from build123d import *

# Parameters (mm, degrees)
CUT_EXTRUDE1_REACH             = 92.696
SKETCH3_R                      = 3.571875
CUT_EXTRUDE1_DIRECTION_2_DEPTH = 91.696141042
SKETCH4_R                      = 4.7625
CUT_EXTRUDE2_DEPTH             = 2.54


with BuildPart() as part:
    # Sketch2 → Revolve1 (revolve)
    with BuildSketch(Plane(origin=(0, 0, 0), x_dir=(0, 0, -1), z_dir=(1, 0, 0)), mode=Mode.PRIVATE) as revolve1_sk:
        Polygon((0, 63.5), (0, 60.325), (6.35, 60.325), (6.35, 0), (12.7, 0), (12.7, 63.5), align=None)
    revolve(revolve1_sk.sketch.rotate(Axis((0, 0, 40.533532934), (0, 0, -1)), 90), axis=Axis((0, 0, 40.533532934), (0, 0, -1)))

    # Sketch3 → Cut-Extrude1 (cut, up to next)
    with BuildSketch(Plane(origin=(0, 0, -12.7), x_dir=(-1, 0, 0), z_dir=(0, 0, -1)), mode=Mode.PRIVATE) as cut_extrude1_sk1:
        with Locations(Location((0, 0, 0), (0, 0, 180))):
            Circle(SKETCH3_R)
    cut_extrude1_tool1 = extrude(cut_extrude1_sk1.sketch, amount=-CUT_EXTRUDE1_REACH, mode=Mode.PRIVATE) & part.part
    add(cut_extrude1_tool1.solids().sort_by_distance((0, 0, -12.7))[0], mode=Mode.SUBTRACT)

    # Sketch3 → Cut-Extrude1 direction 2 (cut)
    with BuildSketch(Plane(origin=(0, 0, -12.7), x_dir=(-1, 0, 0), z_dir=(0, 0, -1))):
        with Locations(Location((0, 0, 0), (0, 0, 180))):
            Circle(SKETCH3_R)
    extrude(amount=CUT_EXTRUDE1_DIRECTION_2_DEPTH, mode=Mode.SUBTRACT)

    # Sketch4 → Cut-Extrude2 (cut)
    with BuildSketch(Plane.XY.offset(-6.35)):
        Circle(SKETCH4_R)
    extrude(amount=-CUT_EXTRUDE2_DEPTH, mode=Mode.SUBTRACT)


solid = part.part
Part model, mm, in its own coordinate system. A direction names the side the tool comes from. Coordinates: 2 decimals unless noted, no trailing zeros. Loops run counter-clockwise (first coordinate to the right, second up) from the corner with the lowest first, then second, coordinate; pieces in that order, holes last. Notation, with made-up numbers: (-38.75, 14.25) - (-9.75, 14.25) arc R19 ccw to (-9.75, 46.25) - close; hole circle Ø5 at (-23, 72.5). An arc over 180 degrees is marked (long way). Write each question's results on one line, items separated by ' | '. Start each with the question number.
Q1. Drop flat-ended pins along their axis: pin 1 Ø6 at (y, z) = (-50.5, -3) entering from +X; pin 2 Ø4 at (y, z) = (45.5, -9.5) entering from -X; pin 3 Ø5 at (x, z) = (-49.5, -7.5) entering from +Y. Give the stop position or say it passes through.
Q2. Slice it at C-C on z = -10.5. Give the cut face in (x, y), and give its area (3 significant figures).
Q3. Which spindle directions (+Z, -Z, +X, -X, +Y, -Y) get a long thin tool onto all of the face, cutting with end or side? Do faces 1 (the cylindrical face through (-13.77, 61.99, -6.26)), 2 (the cylindrical face through (-3.78, -2.9, -7.6)). Say none if no direction does.
Q4. Probe line 1 along Y through (x, z) = (0, -7.6); line 2 along Y through (x, z) = (0, -2.25) (3 decimals); line 3 along Z through (x, y) = (-31.5, 22). List the from-to ranges inside material, lowest first.
Q5. Slice it at D-D on x = -35. Give the cut face in (y, z), and give its area (3 significant figures).
Answer:
1) pin 1: stops at x = 42.14 | pin 2: stops at x = -46.26 | pin 3: stops at y = 42.7
2) outline: circle Ø127 at (0, 0); hole circle Ø7.14 at (0, 0) | area: 12,600 mm2
3) face 1: +Z, -Z | face 2: +Z
4) line 1: y = -63.5 to -4.76, 4.76 to 63.5 | line 2: y = -63.5 to -60.325, 60.325 to 63.5 | line 3: z = -12.7 to -6.35
5) outline: (-52.98, -12.7) - (52.98, -12.7) - (52.98, 0) - (49.13, 0) - (49.13, -6.35) - (-49.13, -6.35) - (-49.13, 0) - (-52.98, 0) - close | area: 722 mm2
